Geometry: final body of the model. Coordinates: model frame, mm. A direction names the side the tool comes from. Coordinates: 2 decimals unless noted, no trailing zeros. Write each loop counter-clockwise with the first axis right and the second up, starting at its lowest first coordinate (ties: lowest second). Pieces come first, ordered by that corner, then holes.
Autodesk Inventor part; units mm, degrees
ref_plane "Work Plane1" through (0, 0, 23) normal (0, 0, 1) x (1, 0, 0)
ref_plane "YZ Plane" through (0, 0, 0) normal (1, 0, 0) x (0, 1, 0)
ref_plane "XZ Plane" through (0, 0, 0) normal (0, 1, 0) x (-1, 0, 0)
sketch "Sketch1" plane through (0, 0, 0) normal (0, 1, 0) x (-1, 0, 0)
  circle A0 centre (0, 0) radius 20
  circle A1 centre (0, 0) radius 23
  dimension "d0" = 40
  dimension "d1" = 3
extrude "Extrusion1" add sketch "Sketch1" along normal blind 150
ref_plane "Work Plane1" through (0, 0, 23) normal (0, 0, 1) x (1, 0, 0)
sketch "Sketch2" plane through (0, 0, 23) normal (0, 0, 1) x (1, 0, 0)
  line L0 (-17.5, 140) -> (17.5, 140)
  line L1 (17.5, 140) -> (17.5, 105)
  line L2 (17.5, 105) -> (-17.5, 105)
  line L3 (-17.5, 105) -> (-17.5, 140)
  line L4 (-17.5, 90) -> (17.5, 90)
  line L5 (17.5, 90) -> (17.5, 55)
  line L6 (17.5, 55) -> (-17.5, 55)
  line L7 (-17.5, 55) -> (-17.5, 90)
  line L8 (23, 150) -> (-23, 150)
  line L9 (0, 156) -> (0, -26)
  line L10 (-23, 0) -> (23, 0)
  point P0 (0, 0)
  dimension "d5" = 10
  dimension "d6" = 35
  dimension "d7" = 17.5
  dimension "d8" = 35
  dimension "d9" = 35
  dimension "d23" = 15
  dimension "d24" = 55
extrude "Extrusion2" [suppressed]
fillet "Fillet1" [suppressed]
sketch "Sketch3" plane through (0, 0, 0) normal (0, 0, 1) x (1, 0, 0)
  line L0 (23, 150) -> (-23, 150)
  point P0 (0, 0)
  point P1 (0, 100)
  point P2 (0, 70)
  dimension "d14" = 30
  dimension "d15" = 50
hole "Hole1" at (0, 100, 0) at (0, 70, 0) direction (0, 0, -1) diameter 4.5 end through all
sketch "Sketch4" plane through (0, 150, 0) normal (0, 1, 0) x (1, 0, 0)
  circle A0 centre (0, 0) radius 20
  circle A1 centre (0, 0) radius 23
  line L0 (15, 17.4356) -> (15, -17.4356)
  circle A2 centre (0, 0) radius 23
  dimension "d25" = 15
extrude "Extrusion3" cut sketch "Sketch4" against normal blind 35 contours A0 L0 | A0 L0 A1 picked at (16.6667, 0) picked at (17.0329, 12.1097)
fillet "Fillet2" radius 2 2 edges at (15, 115, -15.3322) (15, 115, 15.3322)
sketch "Sketch5" plane through (0, 0, 0) normal (0, -1, 0) x (1, 0, 0)
  circle A0 centre (0, 0) radius 20
  circle A1 centre (0, 0) radius 23
  line L0 (-22.4499, 5) -> (22.4499, 5)
  circle A2 centre (0, 0) radius 23
  dimension "d29" = 5
extrude "Extrusion4" cut sketch "Sketch5" against normal blind 30 contours L0 A0 | A0 L0 A1 picked at (5.8749, 6.4846) picked at (-0.7969, 21.8366)
fillet "Fillet3" radius 2 2 edges at (-20.9074, 30, 5) (20.9074, 30, 5)
equation "\"d7\" = 0.5 * d6"
equation "\"d8\" = d6"
equation "\"d9\" = d8"
properties part number "Pancake_Drop Pipe" material "PVC-Piping"
Item 1: Set-up query: faces 1 (the cylindrical face through (0.86, 97.92, -21.46)), 2 (the flat face through (21, 14, 5)), 3 (the flat face through (21, 115, 0)). Return all of +Z, -Z, +X, -X, +Y, -Y with unobstructed straight access to the full face (end or side cutting, diameter ignored); none if empty.
Derived:
face 1: -Z
face 2: +Z, +X, -X, -Y
face 3: +Z, -Z, +X, +Y
Item 2: Section A-A, the plane z = 0. Output: boundary loops of the cut face in (x, y), plus the area to 3 significant figures.
Derived:
outline: (-23, 0) - (-20, 0) - (-20, 150) - (-23, 150) - close; (20, 0) - (23, 0) - (23, 115) - (20, 115) - close
area: 795 mm2
Item 3: Pull-direction query (X, two-part tool) for faces 4 (the flat face through (0.1, 0, -20.3)), 5 (the cylindrical face through (-12.365, 73.95, -19.394)), 6 (the flat face through (15, 134, -15)), 7 (the cylindrical face through (0.86, 67.92, -21.46)); classes: released by +X, released by -X, zero draft, split by the parting line, or undercut.
Derived:
face 4: zero draft
face 5: split by the parting line
face 6: released by +X
face 7: undercut
Item 4: Section D-D, the plane y = 74. Output: boundary loops of the cut face in (x, z).
Derived:
outline: circle Ø46 at (0, 0); hole circle Ø40 at (0, 0)
Item 5: Section C-C, the plane x = -15.5. Output: boundary loops of the cut face in (y, z).
Derived:
outline: (0, -16.99) - (150, -16.99) - (150, -12.64) - (0, -12.64) - close; (30, 12.64) - (150, 12.64) - (150, 16.99) - (30, 16.99) - close
Item 6: Material intervals for probe 1 along Y at (x, z) = (0, -21.25); probe 2 along Z at (x, y) = (0, 118), sorted ascending.
Derived:
probe 1: y = 0 to 67.75, 72.25 to 97.75, 102.25 to 150
probe 2: z = -23 to -20, 20 to 23
Item 7: Pin query (flat end, axial travel): pin 1 (5 mm diameter, centred on x = 18.5, z = 3, fed in from +Y); pin 2 (4.5 mm diameter, centred on y = 132.5, z = -15, fed in from +X); pin 3 (1 mm diameter, centred on x = 6, y = 40, fed in from +Z). Return the tip coordinate at first contact, or that it passes through.
Derived:
pin 1: stops at y = 115
pin 2: stops at x = 15
pin 3: stops at z = 22.33
Item 8: Section B-B, the plane x = 0. Output: boundary loops of the cut face in (y, z), plus the area to 3 significant figures.
Derived:
outline: (0, -23) - (67.75, -23) - (67.75, -20) - (0, -20) - close; (30, 20) - (150, 20) - (150, 23) - (30, 23) - close; (72.25, -23) - (97.75, -23) - (97.75, -20) - (72.25, -20) - close; (102.25, -23) - (150, -23) - (150, -20) - (102.25, -20) - close
area: 783 mm2
